Verification items for the finished model (mm, model axes). Give positions to 0.01 mm unless a question says otherwise; leave off trailing zeros. Order: outer loops, then holes, each group sorted by start corner. A loop starts at its lowest first (then second) coordinate and runs counter-clockwise, first axis right, second up. Notation, with made-up numbers: (53.25, 36) - (60.25, 36) arc R11 ccw to (60.25, 55) - close; hole circle Ø10 at (-11.75, -33.75). An arc over 180 degrees is marked (long way). Answer as a JSON object with one key per item and string values.
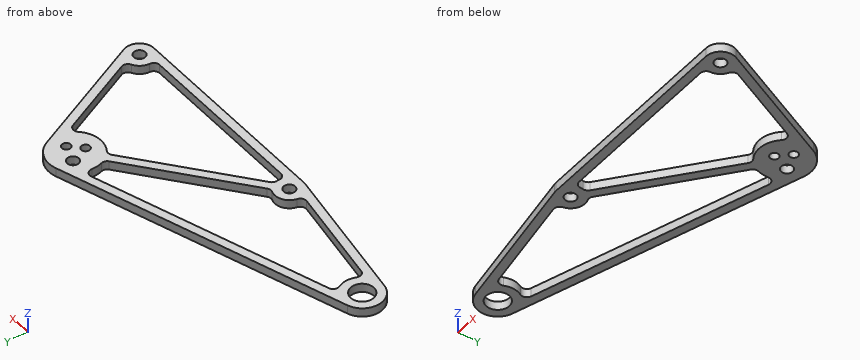
Autodesk Inventor part; units mm, degrees
ref_plane "YZ Plane" through (0, 0, 0) normal (1, 0, 0) x (0, 1, 0)
ref_plane "XZ Plane" through (0, 0, 0) normal (0, 1, 0) x (-1, 0, 0)
ref_plane "XY Plane" through (0, 0, 0) normal (0, 0, 1) x (1, 0, 0)
sketch "スケッチ1" plane through (0, 0, 0) normal (0, 0, 1) x (1, 0, 0)
  circle A0 centre (-11.4931, -19.1593) radius 14 construction
  circle A1 centre (16.245, -15.3385) radius 14 construction
  line L0 (-170.915, -81.4118) -> (490.0044, -81.4118)
  line L1 (-197.2268, -33.1593) -> (179.6604, -33.1593) construction
  line L2 (-178.6504, 68.5882) -> (447.0756, 68.5882) construction
  circle A2 centre (-11.4931, -19.1593) radius 14 construction
  circle A3 centre (-21.8854, 6.8407) radius 14 construction
  circle A4 centre (-0.5211, 0.3031) radius 20.05 construction
  circle A5 centre (-0.5211, 0.3031) radius 22.3421 construction
  circle A6 centre (0, 0) radius 22.3421 construction
  circle A7 centre (-0.5211, 0.3031) radius 5.05 construction
  circle A8 centre (19.689, 29.6103) radius 30.55 construction
  circle A9 centre (19.689, 29.6103) radius 10.1 construction
  circle A10 centre (39.672, 58.5882) radius 25.1 construction
  line L3 (-0.5211, 0.3031) -> (39.672, 58.5882) construction
  circle A11 centre (39.672, 58.5882) radius 27.1 construction
  circle A12 centre (19.689, 29.6103) radius 31.55 construction
  circle A13 centre (19.689, 29.6103) radius 12.1 construction
  circle A14 centre (-0.5211, 0.3031) radius 20.55 construction
  circle A15 centre (-0.5211, 0.3031) radius 6.05 construction
  circle A16 centre (36.8436, 61.4166) radius 4 construction
  circle A17 centre (36.8436, 61.4166) radius 2
  line L4 (36.8436, 61.4166) -> (39.672, 58.5882)
  line L5 (39.672, 58.5882) -> (22.909, 61.4166) construction
  circle A18 centre (22.909, 61.4166) radius 2
  circle A19 centre (22.909, 61.4166) radius 5
  line L6 (28.2635, 50.4737) -> (31.5576, 69.9968) construction
  line L7 (31.5576, 69.9968) -> (51.0806, 66.7027) construction
  line L8 (51.0806, 66.7027) -> (47.7865, 47.1796) construction
  line L9 (47.7865, 47.1796) -> (28.2635, 50.4737) construction
  circle A20 centre (39.672, 58.5882) radius 9
  circle A21 centre (28.2635, 50.4737) radius 2.5
  circle A22 centre (47.7865, 47.1796) radius 2.5
  circle A23 centre (51.0806, 66.7027) radius 2.5
  circle A24 centre (31.5576, 69.9968) radius 2.5
  circle A25 centre (28.2635, 50.4737) radius 5
  line L10 (22.909, 61.4166) -> (36.8436, 61.4166) construction
  line L11 (-26.0808, 51.4166) -> (-426.0808, 51.4166)
  line L12 (-26.0808, 24.4166) -> (23.9192, 24.4166)
  circle A26 centre (39.672, 58.5882) radius 17.5
  circle A27 centre (47.7865, 47.1796) radius 2.1
  circle A28 centre (28.2635, 50.4737) radius 2.1
  circle A29 centre (31.5576, 69.9968) radius 2.1
  circle A30 centre (51.0806, 66.7027) radius 2.1
  circle A31 centre (47.7865, 47.1796) radius 5
  circle A32 centre (31.5576, 69.9968) radius 5
  circle A33 centre (51.0806, 66.7027) radius 5
  circle A34 centre (39.672, 58.5882) radius 19.5
  circle A35 centre (39.672, 58.5882) radius 20.5
  line L13 (20.7504, 89.6882) -> (53.4998, 89.6882)
  line L14 (53.4998, 89.6882) -> (73.6516, 68.9857)
  line L15 (20.7504, 89.6882) -> (-13.977, 39.0272)
  circle A36 centre (-59.2702, 32.0272) radius 5.025 construction
  circle A37 centre (-59.2702, 32.0272) radius 4
  arc A38 (-59.2702, 39.0272) -> (-62.5897, 25.8643) centre (-59.2702, 32.0272) ccw
  line L16 (-59.2702, 39.0272) -> (-13.977, 39.0272)
  line L17 (-62.5897, 25.8643) -> (-36.5547, 11.8407)
  line L18 (-36.5547, 11.8407) -> (-36.5547, -33.1593)
  arc A39 (74.5655, 64.0796) -> (73.6516, 68.9857) centre (70.4271, 65.8469) ccw
  circle A40 centre (8.5193, 63.8863) radius 4.5 construction
  arc A41 (59.4085, 28.8085) -> (59.8353, 29.5856) centre (55.6969, 31.3528) ccw
  circle A42 centre (23.6647, -6.2198) radius 4.5
  circle A43 centre (-16.0241, 34.5272) radius 4.5 construction
  line L19 (59.8353, 29.5856) -> (74.5655, 64.0796)
  line L20 (32.172, 89.6882) -> (32.172, 92.6882)
  line L21 (32.172, 92.6882) -> (47.172, 92.6882)
  line L22 (47.172, 92.6882) -> (47.172, 89.6882)
  line L23 (35.172, 89.6882) -> (35.172, 86.6882)
  line L24 (35.172, 86.6882) -> (44.172, 86.6882)
  line L25 (44.172, 86.6882) -> (44.172, 89.6882)
  circle A44 centre (70.4271, 65.8469) radius 1.5
  circle A45 centre (55.6969, 31.3528) radius 1.5
  circle A46 centre (23.6647, -6.2198) radius 1.5
  circle A47 centre (-16.0241, 34.5272) radius 1.5
  circle A48 centre (8.5193, 63.8863) radius 1.5
  circle A49 centre (-10.0662, 20.4166) radius 4 construction
  circle A50 centre (-10.0662, 20.4166) radius 2
  line L26 (1.9305, -36.1593) -> (16.9305, -36.1593)
  line L27 (16.9305, -36.1593) -> (16.9305, -33.1593)
  line L28 (1.9305, -33.1593) -> (1.9305, -36.1593)
  arc A51 (1.9305, -33.1593) -> (-0.1695, -33.1593) centre (0.8805, -33.1593) ccw
  line L29 (13.9305, -30.1593) -> (13.9305, -33.1593)
  arc A52 (13.9305, -30.1593) -> (11.8305, -30.1593) centre (12.8805, -30.1593) ccw
  line L30 (7.0305, -30.1593) -> (11.8305, -30.1593)
  arc A53 (7.0305, -30.1593) -> (4.9305, -30.1593) centre (5.9805, -30.1593) ccw
  line L31 (4.9305, -33.1593) -> (4.9305, -30.1593)
  arc A54 (4.9305, -33.1593) -> (7.0305, -33.1593) centre (5.9805, -33.1593) ccw
  arc A55 (11.8305, -33.1593) -> (13.9305, -33.1593) centre (12.8805, -33.1593) ccw
  line L32 (-36.5547, -36.1593) -> (-21.5547, -36.1593)
  line L33 (-21.5547, -36.1593) -> (-21.5547, -33.1593)
  arc A56 (-19.4547, -33.1593) -> (-21.5547, -33.1593) centre (-20.5047, -33.1593) ccw
  line L34 (-36.5547, -33.1593) -> (-36.5547, -36.1593)
  arc A57 (-33.5547, -33.1593) -> (-31.4547, -33.1593) centre (-32.5047, -33.1593) ccw
  line L35 (-33.5547, -33.1593) -> (-33.5547, -30.1593)
  arc A58 (-31.4547, -30.1593) -> (-33.5547, -30.1593) centre (-32.5047, -30.1593) ccw
  line L36 (-31.4547, -30.1593) -> (-26.6547, -30.1593)
  arc A59 (-24.5547, -30.1593) -> (-26.6547, -30.1593) centre (-25.6047, -30.1593) ccw
  line L37 (-24.5547, -30.1593) -> (-24.5547, -33.1593)
  arc A60 (-26.6547, -33.1593) -> (-24.5547, -33.1593) centre (-25.6047, -33.1593) ccw
  line L38 (59.4085, 28.8085) -> (16.9305, -33.1593)
  circle A61 centre (-21.8854, 6.8407) radius 5
  circle A62 centre (-11.4931, -19.1593) radius 5
  line L39 (-31.4547, -33.1593) -> (-26.6547, -33.1593)
  line L40 (-19.4547, -33.1593) -> (-0.1695, -33.1593)
  line L41 (7.0305, -33.1593) -> (11.8305, -33.1593)
  line L42 (0.4485, -25.8914) -> (-27.1419, -10.3373) construction
  line L43 (-27.1419, -10.3373) -> (-17.3768, 21.5744) construction
  circle A63 centre (-21.8854, 6.8407) radius 8
  circle A64 centre (-11.4931, -19.1593) radius 8
  circle A65 centre (-19.5445, 14.4905) radius 1.3
  circle A66 centre (-24.2262, -0.8092) radius 1.3
  circle A67 centre (-18.4619, -15.2306) radius 1.3
  circle A68 centre (-4.5242, -23.088) radius 1.3
  circle A69 centre (-0.5211, 0.3031) radius 4.5
  circle A70 centre (19.689, 29.6103) radius 6
  arc A71 (65.9325, 14.9991) -> (66.6936, 19.6662) centre (63.1287, 17.8519) ccw
  line L44 (16.9305, -33.1593) -> (65.9325, 14.9991)
  line L45 (66.6936, 19.6662) -> (60.6612, 31.5196)
  circle A72 centre (63.1287, 17.8519) radius 2
  dimension "d0" = 150
  dimension "d1" = 28
  dimension "d2" = 28
  dimension "d3" = 40.1
  dimension "d4" = 10.1
  dimension "d5" = 61.1
  dimension "d6" = 20.2
  dimension "d7" = 50.2
  dimension "d8" = 10
  dimension "d9" = 2
  dimension "d10" = 1
  dimension "d11" = 2
  dimension "d12" = 0.5
  dimension "d13" = 1
  dimension "d14" = 40
  dimension "d15" = 8
  dimension "d16" = 4
  dimension "d17" = 4
  dimension "d18" = 45
  dimension "d19" = 17
  dimension "d20" = 4
  dimension "d21" = 3
  dimension "d22" = 1
  dimension "d23" = 5
  dimension "d24" = 5
  dimension "d25" = 5
  dimension "d26" = 5
  dimension "d27" = 10
  dimension "d28" = 400
  dimension "d29" = 10
  dimension "d30" = 50
  dimension "d31" = 50
  dimension "d32" = 27
  dimension "d33" = 27
  dimension "d34" = 35
  dimension "d35" = 4.2
  dimension "d36" = 4.2
  dimension "d37" = 4.2
  dimension "d38" = 4.2
  dimension "d39" = 10
  dimension "d40" = 10
  dimension "d41" = 10
  dimension "d42" = 2
  dimension "d43" = 1
  dimension "d44" = 8
  dimension "d45" = 3
  dimension "d46" = 4
  dimension "d47" = 9
  dimension "d48" = 9
  dimension "d49" = 9
  dimension "d50" = 9
  dimension "d51" = 9
  dimension "d52" = 3
  dimension "d53" = 15
  dimension "d54" = 3
  dimension "d55" = 9
  dimension "d56" = 3
  dimension "d57" = 7.5
  dimension "d58" = 3
  dimension "d59" = 3
  dimension "d60" = 3
  dimension "d61" = 3
  dimension "d62" = 3
  dimension "d63" = 8
sketch "スケッチ2" plane through (0, 0, 0) normal (0, 0, 1) x (1, 0, 0)
  circle A0 centre (-59.2702, 32.0272) radius 4
  circle A1 centre (63.1287, 17.8519) radius 2
  circle A2 centre (-10.0662, 20.4166) radius 2
  circle A3 centre (36.8436, 61.4166) radius 2
  arc A4 (-61.2167, 38.7511) -> (-60.607, 25.156) centre (-59.2702, 32.0272) ccw
  arc A5 (-11.0211, 15.5087) -> (-10.2413, 15.4197) centre (-10.0662, 20.4166) ccw
  arc A6 (62.9536, 12.855) -> (67.6583, 19.9692) centre (63.1287, 17.8519) ccw
  circle A7 centre (39.672, 58.5882) radius 9
  circle A8 centre (39.672, 58.5882) radius 7 construction
  circle A9 centre (43.1475, 59.0018) radius 1.5
  circle A10 centre (39.2584, 55.1127) radius 1.5
  line L0 (43.1475, 59.0018) -> (39.2584, 55.1127) construction
  line L1 (39.2584, 55.1127) -> (36.8436, 61.4166) construction
  line L2 (36.8436, 61.4166) -> (43.1475, 59.0018) construction
  line L3 (36.8436, 61.4166) -> (41.203, 57.0573) construction
  line L4 (-61.2167, 38.7511) -> (37.1693, 67.2332)
  line L5 (47.8253, 62.3993) -> (67.6583, 19.9692)
  line L6 (62.9536, 12.855) -> (-10.2413, 15.4197)
  line L7 (-11.0211, 15.5087) -> (-60.607, 25.156)
  line L8 (39.672, 58.5882) -> (-10.0662, 20.4166) construction
  line L9 (38.7588, 59.7782) -> (-10.9794, 21.6066)
  line L10 (-9.1529, 19.2267) -> (40.5853, 57.3982)
  arc A11 (40.5853, 57.3982) -> (38.7588, 59.7782) centre (39.672, 58.5882) ccw
  arc A12 (-10.9794, 21.6066) -> (-9.1529, 19.2267) centre (-10.0662, 20.4166) ccw
  line L11 (38.0036, 64.3516) -> (-60.3825, 35.8694)
  arc A13 (-60.3825, 35.8694) -> (-60.0341, 28.1008) centre (-59.2702, 32.0272) ccw
  line L12 (-60.0341, 28.1008) -> (-10.4481, 18.4534)
  arc A14 (-10.4481, 18.4534) -> (-10.1362, 18.4179) centre (-10.0662, 20.4166) ccw
  line L13 (-10.1362, 18.4179) -> (63.0587, 15.8532)
  arc A15 (63.0587, 15.8532) -> (64.9406, 18.6989) centre (63.1287, 17.8519) ccw
  line L14 (64.9406, 18.6989) -> (45.1075, 61.1289)
  circle A16 centre (-59.2702, 32.0272) radius 7
  circle A17 centre (-10.0662, 20.4166) radius 5
  circle A18 centre (63.1287, 17.8519) radius 5
  point P0 (0, 0)
  point P1 (14.8029, 39.5024)
  point P2 (-7.1956, 24.5105)
  point P3 (-14.9464, 19.3286)
  point P4 (-54.3952, 27.0037)
  point P5 (-54.8645, 37.4668)
  point P6 (31.5599, 62.4862)
  point P7 (31.7189, 54.3754)
  point P8 (-5.5565, 18.2574)
  point P9 (-5.3691, 22.1306)
  point P10 (33.5454, 51.9955)
  point P11 (47.9481, 55.0518)
  point P12 (63.0001, 22.8503)
  point P13 (58.4789, 16.0136)
  dimension "d77" = 3
  dimension "d78" = 3
  dimension "d80" = 3
  dimension "d82" = 14
  dimension "d83" = 3
  dimension "d84" = 3
  dimension "d85" = 5.5
  dimension "d86" = 3.5
  dimension "d87" = 3
  dimension "d88" = 3
  dimension "d89" = 3
  dimension "d90" = 3
  dimension "d91" = 3
extrude "押し出し1" add sketch "スケッチ2" along normal blind 3 contours A0 L11 A16 L12 | A0 L12 A16 A4 L11 | A16 L4 A7 L11 | L12 A17 L7 A16 | A7 L10 A10 A11 L9 | A17 L9 A2 L12 | L12 A2 L13 A17 A5 | L9 A11 L10 A10 A7 | A7 L10 A17 L9 | A17 L10 A2 L9 | L5 A18 L14 A7 | A2 L10 A17 L13 | A17 L13 A18 L6 | A6 A18 L13 A1 L14 | L14 A1 L13 A18
fillet "フィレット1" radius 2 12 edges at (-5.5565, 18.2574, 1.5) (-5.3691, 22.1306, 1.5) (58.4789, 16.0136, 1.5) (63.0001, 22.8503, 1.5) (47.9481, 55.0518, 1.5) (33.5454, 51.9955, 1.5) (-7.1956, 24.5105, 1.5) (-14.9464, 19.3286, 1.5) (31.7189, 54.3754, 1.5) (31.5599, 62.4862, 1.5) (-54.8645, 37.4668, 1.5) (-54.3952, 27.0037, 1.5)
properties part number "横回転首振りフレーム３" material "アルミニウム 2014-T4"
(1) Section check B-B (y = 44). Record the cut outline in (x, z).
Computed values:
{"outline": "(-43.09, 0) - (-32.3, 0) - (-32.3, 3) - (-43.09, 3) - close; (18.2, 0) - (23.13, 0) - (23.13, 3) - (18.2, 3) - close; (53.11, 0) - (56.43, 0) - (56.43, 3) - (53.11, 3) - close"}
(2) Section check C-C (x = -32.5). Record the cut outline in (y, z), then the cut area to 3 significant figures.
Computed values:
{"outline": "(19.69, 0) - (22.74, 0) - (22.74, 3) - (19.69, 3) - close; (43.94, 0) - (47.06, 0) - (47.06, 3) - (43.94, 3) - close", "area": "18.5 mm²"}
(3) Section check A-A (x = 23.5). Record the cut outline in (y, z).
Computed values:
{"outline": "(14.24, 0) - (17.24, 0) - (17.24, 3) - (14.24, 3) - close; (44.29, 0) - (48.07, 0) - (48.07, 3) - (44.29, 3) - close; (60.15, 0) - (63.28, 0) - (63.28, 3) - (60.15, 3) - close"}
(4) Section check D-D (z = 0.6). Count the separate pieces of the cut face and the enclosed holes in it, then the cut area to 3 significant figures.
Computed values:
{"separate pieces": "1", "enclosed holes": "8", "area": "1,350 mm²"}
(5) Gauge pin test, flat end, axial feed: pin 1 Ø1 at (x, z) = (46.5, 1.5) entering from +Y. Record the tip position at first contact, or that the pin passes through.
Computed values:
{"pin 1": "stops at y = 64.99"}
(6) Material ranges on line 1 along Y through (x, z) = (24.5, 2.2); line 2 along Y through (x, z) = (42.5, 1.15); line 3 along Y through (x, z) = (-32, 2.8), recorded low to high. Write a range as [from, to].
Computed values:
{"line 1": "y = [14.2, 17.2], [45.05, 48.84], [60.44, 63.57]", "line 2": "y = [13.57, 16.57], [50.04, 57.65], [60.35, 67.13]", "line 3": "y = [19.59, 22.65], [44.09, 47.21]"}
